Source: three-view drawing plus pictorial views. Frame: mm from the lowest corner of the part. A direction names the side the tool comes from. Give positions to 0.01 mm unless a question says otherwise; leave off trailing zeros. Write each loop counter-clockwise with the first axis right and the second up, starting at its lowest first coordinate (ties: lowest second). Pieces come first, ordered by that corner, then holes. Notation, with made-up numbers: M 61.25,30.25 L 70.25,30.25 A18 cw 70.25,46.25 Z; hole C 41.25,-21 d2. An arc over 180 degrees is marked long. Return JSON: item names as keys, results as strings.
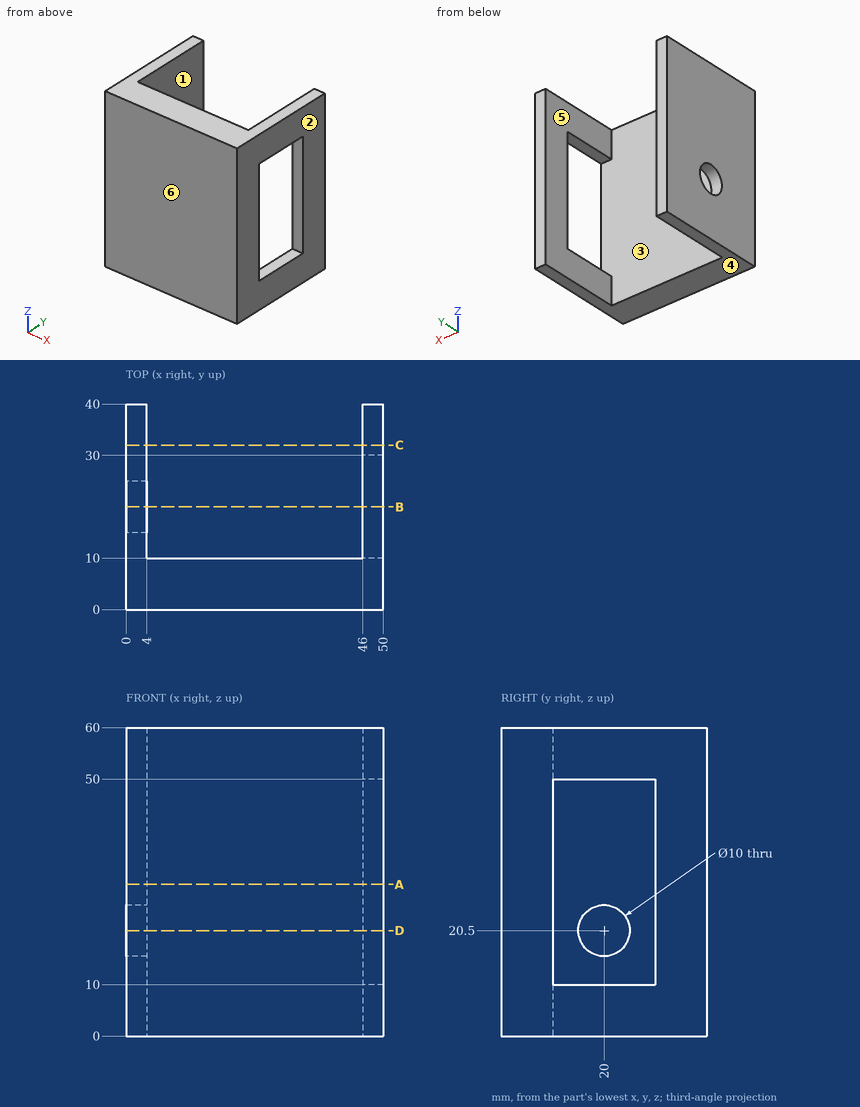
1) Line query: line 1 (Y direction, x = 1.65, z = 20.5); line 2 (X direction, y = 30.5, z = 20); line 3 (Y direction, x = 46.5, z = 37). Output: solid intervals per line, ascending. Write a range as [from, to].
Numbers:
{"line 1": "y = [0, 15], [25, 40]", "line 2": "x = [0, 4], [46, 50]", "line 3": "y = [0, 10], [30, 40]"}
2) Draft query along X for the marked faces 1, 2, 3 and 4. Return one class per face: released by +X, released by -X, zero draft, split by the parting line, or undercut.
Numbers:
{"face 1": "undercut", "face 2": "released by +X", "face 3": "undercut", "face 4": "zero draft"}
3) Cut plane D-D, the plane z = 20.5. Return the cut outline in (x, y).
Numbers:
{"outline": "M 0,0 L 50,0 L 50,10 L 4,10 L 4,15 L 0,15 Z; M 0,25 L 4,25 L 4,40 L 0,40 Z; M 46,30 L 50,30 L 50,40 L 46,40 Z"}
4) Cut plane B-B, the plane y = 20. Return the cut outline in (x, z), then the cut area to 3 significant figures.
Numbers:
{"outline": "M 0,0 L 4,0 L 4,15.5 L 0,15.5 Z; M 0,25.5 L 4,25.5 L 4,60 L 0,60 Z; M 46,0 L 50,0 L 50,10 L 46,10 Z; M 46,50 L 50,50 L 50,60 L 46,60 Z", "area": "280 mm²"}
5) Contact query for flat-ended pins moving along their axis: pin 1 Ø8 at (y, z) = (20, 20.5) entering from -X; pin 2 Ø1 at (x, z) = (33, 41.5) entering from +Y; pin 3 Ø3 at (y, z) = (17.5, 40) entering from +X. Output: stop coordinate, or through.
Numbers:
{"pin 1": "passes through", "pin 2": "stops at y = 10", "pin 3": "stops at x = 4"}
6) Cut plane A-A, the plane z = 29.5. Return the cut outline in (x, y), then the cut area to 3 significant figures.
Numbers:
{"outline": "M 0,0 L 50,0 L 50,10 L 4,10 L 4,40 L 0,40 Z; M 46,30 L 50,30 L 50,40 L 46,40 Z", "area": "660 mm²"}
7) Set-up query: the marked faces 5 and 6. Return all of +Z, -Z, +X, -X, +Y, -Y with unobstructed straight access to the full face (end or side cutting, diameter ignored); none if empty.
Numbers:
{"face 5": "+Z, -Z, +Y", "face 6": "+Z, -Z, +X, -X, -Y"}
8) Cut plane C-C, the plane y = 32. Return the cut outline in (x, z), then the cut area to 3 significant figures.
Numbers:
{"outline": "M 0,0 L 4,0 L 4,60 L 0,60 Z; M 46,0 L 50,0 L 50,60 L 46,60 Z", "area": "480 mm²"}
